CAD build for the part. Positions are in the model's coordinates, mm. A direction names the side the tool comes from. Coordinates: 2 decimals unless noted, no trailing zeros. Order: outer loops, then holes, each group sorted by start corner. A loop starts at its lowest first (then second) coordinate and runs counter-clockwise, first axis right, second up.
from build123d import *

# Parameters (mm, degrees)
SCHNITT_LINEAR_START            = -1
SCHNITT_LINEAR_AUSTRAGEN1_DEPTH = 1
LINEAR_AUSTRAGEN1_DEPTH         = 5


with BuildPart() as part:
    # Skizze2 → Rotation1 (revolve)
    with BuildSketch(Plane.XY, mode=Mode.PRIVATE) as rotation1_sk:
        with BuildLine():
            Line((0, 0), (-1.75, 0))
            Line((-1.75, 0), (-1.75, 0.5))
            Line((-1.75, 0.5), (-1.5, 0.5))
            Line((-1.5, 0.5), (-1.5, 3))
            ThreePointArc((-1.5, 3), (-1.060660172, 4.060660172), (0, 4.5))
            Line((0, 4.5), (0, 0))
        make_face()
    revolve(rotation1_sk.sketch.rotate(Axis((0, 0, 0), (0, 1, 0)), 270), axis=Axis((0, 0, 0), (0, 1, 0)))

    # Skizze3 → Schnitt-Linear austragen1 (cut)
    with BuildSketch(Plane.XZ.offset(SCHNITT_LINEAR_START)):
        with BuildLine():
            Line((1.58113883, -0.75), (1.58113883, 0.75))
            ThreePointArc((1.58113883, 0.75), (1.75, 0), (1.58113883, -0.75))
        make_face()
    extrude(amount=SCHNITT_LINEAR_AUSTRAGEN1_DEPTH, mode=Mode.SUBTRACT)

    # Skizze4 → Linear austragen1 (add)
    with BuildSketch(Plane.XZ):
        with BuildLine():
            Line((0.6, 0.15), (0.8, 0.15))
            ThreePointArc((0.8, 0.15), (0.870710678, 0.120710678), (0.9, 0.05))
            Line((0.9, 0.05), (0.9, -0.05))
            ThreePointArc((0.9, -0.05), (0.870710678, -0.120710678), (0.8, -0.15))
            Line((0.8, -0.15), (0.6, -0.15))
            ThreePointArc((0.6, -0.15), (0.529289322, -0.120710678), (0.5, -0.05))
            Line((0.5, -0.05), (0.5, 0.05))
            ThreePointArc((0.5, 0.05), (0.529289322, 0.120710678), (0.6, 0.15))
        make_face()
        with BuildLine():
            Line((-0.9, 0.15), (-0.6, 0.15))
            ThreePointArc((-0.6, 0.15), (-0.529289322, 0.120710678), (-0.5, 0.05))
            Line((-0.5, 0.05), (-0.5, -0.05))
            ThreePointArc((-0.5, -0.05), (-0.529289322, -0.120710678), (-0.6, -0.15))
            Line((-0.6, -0.15), (-0.9, -0.15))
            ThreePointArc((-0.9, -0.15), (-0.970710678, -0.120710678), (-1, -0.05))
            Line((-1, -0.05), (-1, 0.05))
            ThreePointArc((-1, 0.05), (-0.970710678, 0.120710678), (-0.9, 0.15))
        make_face()
    extrude(amount=LINEAR_AUSTRAGEN1_DEPTH)


solid = part.part
1) Slice it at D-D (y = 3.75). List the corners of the cut face in (x, z), plus the area to 3 significant figures.
2) Slice it at A-A (y = -4). List the corners of the cut face in (x, z).
3) Slice it at B-B (x = 0). List the corners of the cut face in (y, z), plus the area to 3 significant figures.
4) Drill centre lines: probe 1 along X at (y, z) = (-4, -0.05); probe 2 along Y at (x, z) = (-1.3, 0.85); probe 3 along Z at (x, y) = (1.3, 1.75). Where is each one in solid material? Low to high.
5) Slice it at C-C (z = 1.2). List the corners of the cut face in (x, y), plus the area to 3 significant figures.
6) Which spindle directions (+Z, -Z, +X, -X, +Y, -Y) get a long thin tool onto all of the face, cutting with end or side? Do faces 1 (the cylindrical face through (-0.45, 1.77, -1.43)), 2 (the cylindrical face through (-1.75, 0.25, -0.07)). Say none if no direction does.
7) Pin check, flat tips, straight feed: P1, Ø1.5, axis at x = 0, y = -2.5, coming from the +Z side; P2, Ø1, axis at x = 0, z = -1.5, coming from the -Y side. Stop position of each tip, or through.
Worked out:
1. outline: circle Ø2.6 at (0, 0)
1. area: 5.30 mm2
2. outline: (-1, -0.05) arc R0.1 ccw to (-0.9, -0.15) - (-0.6, -0.15) arc R0.1 ccw to (-0.5, -0.05) - (-0.5, 0.05) arc R0.1 ccw to (-0.6, 0.15) - (-0.9, 0.15) arc R0.1 ccw to (-1, 0.05) - close; (0.5, -0.05) arc R0.1 ccw to (0.6, -0.15) - (0.8, -0.15) arc R0.1 ccw to (0.9, -0.05) - (0.9, 0.05) arc R0.1 ccw to (0.8, 0.15) - (0.6, 0.15) arc R0.1 ccw to (0.5, 0.05) - close
3. outline: (0, -1.75) - (0.5, -1.75) - (0.5, -1.5) - (3, -1.5) arc R1.5 ccw to (3, 1.5) - (0.5, 1.5) - (0.5, 1.75) - (0, 1.75) - close
3. area: 12.8 mm2
4. probe 1: x = -1 to -0.5, 0.5 to 0.9
4. probe 2: y = 0 to 0.5
4. probe 3: z = -0.75 to 0.75
5. outline: (-1.27, 0) - (1.27, 0) - (1.27, 0.5) - (0.9, 0.5) - (0.9, 3) arc R0.9 ccw to (-0.9, 3) - (-0.9, 0.5) - (-1.27, 0.5) - close
5. area: 7.05 mm2
6. face 1: +Y
6. face 2: +Y, -Y
7. P1: stops at z = 0.15
7. P2: stops at y = 0
